from build123d import *

# Parameters (mm, degrees)
SKETCH1_W           = 177.8
SKETCH1_H           = 50.8
BOSS_EXTRUDE1_DEPTH = 12.7
SKETCH2_W           = 25.4
SKETCH2_H           = 12.7
SKETCH2_W_2         = 12.7
SKETCH2_H_2         = 25.4
BOSS_EXTRUDE2_DEPTH = 12.7


with BuildPart() as part:
    # Sketch1 → Boss-Extrude1 (new body)
    with BuildSketch(Plane.XY):
        with Locations((-88.9, 25.4)):
            Rectangle(SKETCH1_W, SKETCH1_H)
    extrude(amount=BOSS_EXTRUDE1_DEPTH)

    # Sketch2 → Boss-Extrude2 (add, through all)
    with BuildSketch(Plane.XY.offset(12.7)):
        with Locations((-152.4, 57.15)):
            Rectangle(SKETCH2_W, SKETCH2_H)
        with Locations((-110.066666667, 57.15)):
            Rectangle(SKETCH2_W, SKETCH2_H)
        with Locations((-67.733333333, 57.15)):
            Rectangle(SKETCH2_W, SKETCH2_H)
        with Locations((-25.4, 57.15)):
            Rectangle(SKETCH2_W, SKETCH2_H)
        with Locations((6.35, 25.4)):
            Rectangle(SKETCH2_W_2, SKETCH2_H_2)
        with Locations((-184.15, 25.4)):
            Rectangle(SKETCH2_W_2, SKETCH2_H_2)
    extrude(amount=-BOSS_EXTRUDE2_DEPTH)


solid = part.part
For this review, take the finished solid that the model builds, in its own axes (mm). A direction names the side the tool comes from. Give positions to 0.01 mm unless a question says otherwise; leave off trailing zeros. Loops run counter-clockwise (first coordinate to the right, second up) from the corner with the lowest first, then second, coordinate; pieces in that order, holes last.
Item 1: Take a section at B-B, the plane z = 8.5. State the section outline as (x, y) points.
Item 2: For line 1 along X through (y, z) = (61, 4); line 2 along Y through (x, z) = (-42, 2.25); line 3 along X through (y, z) = (10, 2), list the stretches that pass through material, from the lowest coordinate up.
Item 3: Insertion check: pin 1 (4 mm diameter, centred on y = 56.5, z = 5, fed in from +X); pin 2 (4 mm diameter, centred on x = -4.5, z = 6.5, fed in from +Y); pin 3 (4 mm diameter, centred on y = 59.5, z = 8.5, fed in from -X). Each pin has a flat end and moves straight along its axis. Give the tip position at first contact, or say it passes through.
Item 4: Take a section at D-D, the plane y = 9.5. State the section outline as (x, z) points, and give its area (3 significant figures).
Item 5: Take a section at A-A, the plane y = 54. State the section outline as (x, z) points, and give its area (3 significant figures).
Item 6: Tool access review of faces 4 (the flat face through (6, 38.1, 6)), 5 (the flat face through (-47, 50.8, 6)), 6 (the flat face through (-177.8, 6, 6)): name each direction out of +Z, -Z, +X, -X, +Y, -Y from which nothing blocks a thin tool from reaching the whole face with its end or side.
Item 7: Draft analysis for pull direction X (two halves, no side actions). For faces 1 (the flat face through (-165.1, 57, 6)), 2 (the flat face through (-38.1, 57, 6)), 3 (the flat face through (-184, 12.7, 6)), state which applies: +X half, -X half, draft (parallel to the pull), parting line (faces both ways), or undercut.
Item 8: Take a section at C-C, the plane x = -5.5. State the section outline as (y, z) points.
Calculated:
1. outline: (-190.5, 12.7) - (-177.8, 12.7) - (-177.8, 0) - (0, 0) - (0, 12.7) - (12.7, 12.7) - (12.7, 38.1) - (0, 38.1) - (0, 50.8) - (-12.7, 50.8) - (-12.7, 63.5) - (-38.1, 63.5) - (-38.1, 50.8) - (-55.03, 50.8) - (-55.03, 63.5) - (-80.43, 63.5) - (-80.43, 50.8) - (-97.37, 50.8) - (-97.37, 63.5) - (-122.77, 63.5) - (-122.77, 50.8) - (-139.7, 50.8) - (-139.7, 63.5) - (-165.1, 63.5) - (-165.1, 50.8) - (-177.8, 50.8) - (-177.8, 38.1) - (-190.5, 38.1) - close
2. line 1: x = -165.1 to -139.7, -122.77 to -97.37, -80.43 to -55.03, -38.1 to -12.7
2. line 2: y = 0 to 50.8
2. line 3: x = -177.8 to 0
3. pin 1: stops at x = -12.7
3. pin 2: stops at y = 50.8
3. pin 3: stops at x = -165.1
4. outline: (-177.8, 0) - (0, 0) - (0, 12.7) - (-177.8, 12.7) - close
4. area: 2,260 mm2
5. outline: (-165.1, 0) - (-139.7, 0) - (-139.7, 12.7) - (-165.1, 12.7) - close; (-122.77, 0) - (-97.37, 0) - (-97.37, 12.7) - (-122.77, 12.7) - close; (-80.43, 0) - (-55.03, 0) - (-55.03, 12.7) - (-80.43, 12.7) - close; (-38.1, 0) - (-12.7, 0) - (-12.7, 12.7) - (-38.1, 12.7) - close
5. area: 1,290 mm2
6. face 4: +Z, -Z, +X, +Y
6. face 5: +Z, -Z, +Y
6. face 6: +Z, -Z, -X, -Y
7. face 1: -X half
7. face 2: undercut
7. face 3: draft
8. outline: (0, 0) - (50.8, 0) - (50.8, 12.7) - (0, 12.7) - close
